Autodesk Inventor part; units mm, degrees
ref_plane "YZ Plane" through (0, 0, 0) normal (1, 0, 0) x (0, 1, 0)
ref_plane "XZ Plane" through (0, 0, 0) normal (0, 1, 0) x (-1, 0, 0)
ref_plane "XY Plane" through (0, 0, 0) normal (0, 0, 1) x (1, 0, 0)
sketch "Sketch1" plane through (0, 0, 0) normal (0, 1, 0) x (-1, 0, 0)
  line L0 (-18, 35) -> (18, 35)
  line L1 (18, 35) -> (18, -35)
  line L2 (18, -35) -> (-18, -35)
  line L3 (-18, -35) -> (-18, 35)
  line L4 (-18, 35) -> (18, -35) construction
  line L5 (18, 35) -> (-18, -35) construction
  point P0 (0, 0)
  dimension "d0" = 70
  dimension "d1" = 36
extrude "Extrusion1" add sketch "Sketch1" along normal blind 1.5
sketch "Sketch2" plane through (0, 1.5, 0) normal (0, 1, 0) x (1, 0, 0)
  line L0 (-48.0959, 5) -> (45.6433, 5) construction
  line L1 (-14, -63.3043) -> (-14, 77.913) construction
  line L2 (14, -60.8696) -> (14, 81.5652) construction
  line L3 (-37.753, -31) -> (38.247, -31) construction
  line L4 (0, 110.5391) -> (0, -92.2783) construction
  circle A0 centre (-14, -31) radius 1.5
  circle A1 centre (14, -31) radius 1.5
  circle A2 centre (-14, 5) radius 1.5
  line L5 (-18, -35) -> (18, -35)
  point P0 (0, 0)
  dimension "d4" = 28
  dimension "d5" = 36
  dimension "d6" = 14
  dimension "d7" = 3
  dimension "d8" = 3
  dimension "d9" = 3
  dimension "d10" = 4
extrude "Extrusion2" cut sketch "Sketch2" against normal through all
sketch "Sketch3" plane through (0, 1.5, 0) normal (0, 1, 0) x (1, 0, 0)
  line L0 (-8.1133, -28.6264) -> (5.8867, -28.6264)
  line L1 (5.8867, -28.6264) -> (5.8867, 12.3736)
  line L2 (5.8867, 12.3736) -> (-8.1133, 12.3736)
  line L3 (-8.1133, 12.3736) -> (-8.1133, -28.6264)
  point P0 (0, 0)
  dimension "d13" = 41
  dimension "d14" = 14
extrude "Extrusion3" add sketch "Sketch3" along normal blind 11
sketch "Sketch4" plane through (0, 1.5, 0) normal (0, 1, 0) x (1, 0, 0)
  line L0 (-14.9852, 30) -> (15.0148, 30)
  line L1 (15.0148, 30) -> (15.0148, 60)
  line L2 (15.0148, 60) -> (-14.9852, 60)
  line L3 (-14.9852, 60) -> (-14.9852, 30)
  line L4 (18, 35) -> (-18, 35) construction
  point P0 (0, 0)
  dimension "d17" = 30
  dimension "d18" = 30
  dimension "d21" = 5
extrude "Extrusion4" add sketch "Sketch4" along normal blind 15
properties part number "newhub"
Verification items for the finished model (mm, model axes). A direction names the side the tool comes from. Coordinates: 2 decimals unless noted, no trailing zeros. Order: outer loops, then holes, each group sorted by start corner. A loop starts at its lowest first (then second) coordinate and runs counter-clockwise, first axis right, second up. Notation, with made-up numbers: (25, -3.5) -> (76, -3.5) arc R11 cw to (76, 0.5) -> close; hole circle Ø11 at (-3.75, 45.5). An arc over 180 degrees is marked (long way). Use CSV: the item, a comma, the result in double quotes. Start each with the question number.
Q1. Tool access check on faces 4 (the flat face through (0, 9, -30)), 5 (the flat face through (15.015, 9, -45)), 6 (the flat face through (-1, 7, 28.626)), 7 (the flat face through (-8.113, 7, 8)). Record the directions out of +Z, -Z, +X, -X, +Y, -Y that give a thin tool (end or side, any length) a straight path to the whole face; none if there is none.
Q2. Section check B-B, the plane y = 9. Record the cut outline in (x, z).
Q3. Draft check along X on faces 1 (the flat face through (0, 16.5, -45)), 2 (the flat face through (5.887, 7, 8)), 3 (the cylindrical face through (-15.5, 0.76, -5.07)). Enter one of: +X half, -X half, draft (parallel to the pull), parting line (faces both ways), or undercut.
Q4. Section check C-C, the plane x = -14. Record the cut outline in (y, z).
Q5. Section check D-D, the plane z = 31. Record the cut outline in (x, y).
Q6. Depth check by flat-ended pin: P1, Ø3.5, axis at x = 14, z = 31, coming from the +Y side; P2, Ø7.5, axis at y = 8, z = -46, coming from the +X side; P3, Ø5, axis at x = -3, y = 14.5, coming from the +Z side. Enter the tip coordinate at first touch or a pass-through.
Q7. Thickness scan on line 1 along X through (y, z) = (0.4, 31); line 2 along X through (y, z) = (0.75, -5); line 3 along Z through (x, y) = (-14, 0.95). Record the ranges inside material, lowest first.
Q8. Section check A-A, the plane z = -5. Record the cut outline in (x, y).
Returned:
1,face 4,"+X, -X, +Y"
1,face 5,"+Z, -Z, +X, +Y"
1,face 6,"+Z, +X, -X, +Y"
1,face 7,"+Z, -X, +Y"
2,outline,"(-14.99, -60) -> (15.01, -60) -> (15.01, -30) -> (-14.99, -30) -> close; (-8.11, -12.37) -> (5.89, -12.37) -> (5.89, 28.63) -> (-8.11, 28.63) -> close"
3,face 1,"draft"
3,face 2,"+X half"
3,face 3,"undercut"
4,outline,"(0, -35) -> (1.5, -35) -> (1.5, -60) -> (16.5, -60) -> (16.5, -30) -> (1.5, -30) -> (1.5, -6.5) -> (0, -6.5) -> close; (0, -3.5) -> (1.5, -3.5) -> (1.5, 29.5) -> (0, 29.5) -> close; (0, 32.5) -> (1.5, 32.5) -> (1.5, 35) -> (0, 35) -> close"
5,outline,"(-18, 0) -> (-15.5, 0) -> (-15.5, 1.5) -> (-18, 1.5) -> close; (-12.5, 0) -> (12.5, 0) -> (12.5, 1.5) -> (-12.5, 1.5) -> close; (15.5, 0) -> (18, 0) -> (18, 1.5) -> (15.5, 1.5) -> close"
6,P1,"stops at y = 1.5"
6,P2,"stops at x = 15.01"
6,P3,"stops at z = 28.63"
7,line 1,"x = -18 to -15.5, -12.5 to 12.5, 15.5 to 18"
7,line 2,"x = -18 to -15.5, -12.5 to 18"
7,line 3,"z = -35 to -6.5, -3.5 to 29.5, 32.5 to 35"
8,outline,"(-18, 0) -> (-15.5, 0) -> (-15.5, 1.5) -> (-18, 1.5) -> close; (-12.5, 0) -> (18, 0) -> (18, 1.5) -> (5.89, 1.5) -> (5.89, 12.5) -> (-8.11, 12.5) -> (-8.11, 1.5) -> (-12.5, 1.5) -> close"
